Source: CAD feature listing. Evaluate the final solid. Frame: model axes, mm. Give positions to 0.01 mm unless a question says otherwise; leave off trailing zeros. Loops run counter-clockwise (first coordinate to the right, second up) from the corner with the lowest first, then second, coordinate; pieces in that order, holes last. Notation, with made-up numbers: (-34, 72) -> (4, 72) arc R19 ccw to (4, 80) -> close; hole circle Ø7 at (7.5, 20.25). An arc over 180 degrees is marked (long way). Put each result on its own line as item: value.
```python
from build123d import *

# Parameters (mm, degrees)
SKETCH_1_R      = 3
EXTRUDE_1_DEPTH = 320
CHAMFER_1_SIZE  = 1
CHAMFER_2_SIZE  = 1


with BuildPart() as part:
    # Эскиз1 → Бобышка-Вытянуть1 (new body)
    with BuildSketch(Plane(origin=(0, 0, 0), x_dir=(1, 0, 0), z_dir=(0, 1, 0))):
        Circle(SKETCH_1_R)
    extrude(amount=EXTRUDE_1_DEPTH)

    # Фаска1
    chamfer_1_edges = [part.edges().sort_by_distance(p)[0] for p in [
        (-3, 320, 0),
    ]]
    chamfer(chamfer_1_edges, length=CHAMFER_1_SIZE)

    # Фаска2
    chamfer_2_edges = [part.edges().sort_by_distance(p)[0] for p in [
        (-3, 0, 0),
    ]]
    chamfer(chamfer_2_edges, length=CHAMFER_2_SIZE)


solid = part.part
```
(1) Section A-A on y = 40.5. Return loops of the section in (x, z), then the cut area to 3 significant figures.
Calculated:
outline: circle Ø6 at (0, 0)
area: 28.3 mm²
(2) First-contact query: P1, Ø1, axis at y = 155, z = 1, coming from the -X side; P2, Ø1.5, axis at x = -1, y = 159, coming from the +Z side. Flat tips, straight axial feed; report the tip coordinate or a pass-through.
Calculated:
P1: stops at x = -2.96
P2: stops at z = 2.99
(3) Line query: probe 1 along X at (y, z) = (183, -0.5); probe 2 along Z at (x, y) = (0.3, 37.5); probe 3 along Z at (x, y) = (-0.6, 105). Output: solid intervals per line, ascending. Write a range as from..to.
Calculated:
probe 1: x = -2.96..2.96
probe 2: z = -2.98..2.98
probe 3: z = -2.94..2.94
